Geometry check sheet. Reference: drawing and pictorial views, mm from the part's lowest x, y, z. A direction names the side the tool comes from. Round coordinates to 2 decimals unless told otherwise and drop trailing zeros. Loops run counter-clockwise (first coordinate to the right, second up) from the corner with the lowest first, then second, coordinate; pieces in that order, holes last. Notation, with made-up numbers: M 83.25,-25 L 138.25,-25 A22 cw 138.25,13 Z; hole C 41,-6.75 d7. An arc over 180 degrees is marked long. One line per question, with ' | ' between items. Start each with the question number.
(1) Tool access check on the marked faces 4 and 5. Record the directions out of +Z, -Z, +X, -X, +Y, -Y that give a thin tool (end or side, any length) a straight path to the whole face; none if there is none.
(2) Section check A-A (z = 22). Record the boundary of the cut face in (x, y).
(3) Thickness scan on probe 1 along X at (y, z) = (2.8, 10). Record the ranges inside material, lowest first. Write a range as [from, to].
(4) Section check B-B (y = 0.45). Record the boundary of the cut face in (x, z).
(5) Section check C-C (x = 17.75). Record the boundary of the cut face in (y, z), and give its area (3 significant figures).
(6) Go/stop test with a flat-tipped pin: P1, Ø1.5, axis at x = 6.5, z = 9, coming from the +Y side (1 decimal). Record where the tip stops, or that it passes through.
(7) Draft check along Z on the marked faces 1, 2 and 3. Enter one of: +Z half, -Z half, draft (parallel to the pull), parting line (faces both ways), or undercut.
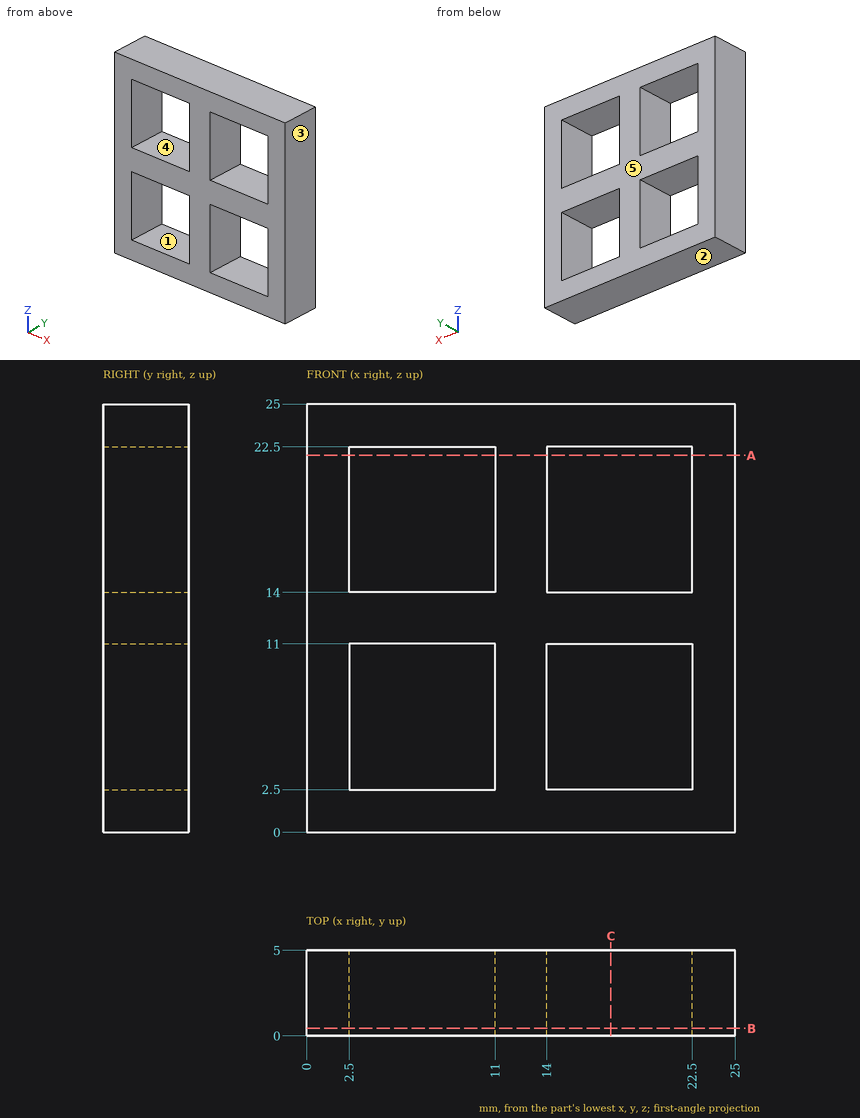
The answers:
1) face 4: +Y, -Y | face 5: +Z, -Z, +X, -X, +Y
2) outline: M 0,0 L 2.5,0 L 2.5,5 L 0,5 Z; M 11,0 L 14,0 L 14,5 L 11,5 Z; M 22.5,0 L 25,0 L 25,5 L 22.5,5 Z
3) probe 1: [0, 2.5], [11, 14], [22.5, 25]
4) outline: M 0,0 L 25,0 L 25,25 L 0,25 Z; hole M 2.5,2.5 L 11,2.5 L 11,11 L 2.5,11 Z; hole M 2.5,14 L 11,14 L 11,22.5 L 2.5,22.5 Z; hole M 14,2.5 L 22.5,2.5 L 22.5,11 L 14,11 Z; hole M 14,14 L 22.5,14 L 22.5,22.5 L 14,22.5 Z
5) outline: M 0,0 L 5,0 L 5,2.5 L 0,2.5 Z; M 0,11 L 5,11 L 5,14 L 0,14 Z; M 0,22.5 L 5,22.5 L 5,25 L 0,25 Z | area: 40.0 mm²
6) P1: through
7) face 1: undercut | face 2: -Z half | face 3: draft
